Design review of the part built by this model. Coordinates are the model's own, in mm. A direction names the side the tool comes from. Give positions to 0.01 mm unless a question says otherwise; leave off trailing zeros. Order: outer loops, then holes, each group sorted by start corner. A loop starts at its lowest first (then second) coordinate and runs counter-clockwise, first axis right, second up. Notation, with made-up numbers: (-8.75, 82) -> (9.25, 82) arc R25 cw to (9.25, 119) -> close; hole circle Ø5 at (-1, 73.25). An arc over 180 degrees is marked (long way). Return JSON: item names as keys, results as strings.
```python
from build123d import *

# Parameters (mm, degrees)
SKETCH1_R           = 4.7625
SKETCH1_R_2         = 3.175
BOSS_EXTRUDE1_DEPTH = 8.3312
BOSS_EXTRUDE2_DEPTH = 8.3312
SKETCH3_R           = 2.0875
SKETCH3_R_2         = 1.5875
BOSS_EXTRUDE3_DEPTH = 8.3312
SKETCH4_R           = 2.0875
BOSS_EXTRUDE4_DEPTH = 0.001
SKETCH5_R           = 1.78
SKETCH5_R_2         = 1.28
BOSS_EXTRUDE5_DEPTH = 11.5062


with BuildPart() as part:
    # Sketch1 → Boss-Extrude1 (new body)
    with BuildSketch(Plane(origin=(0, 0, 0), x_dir=(1, 0, 0), z_dir=(0, 1, 0))):
        with Locations(Location((0, 0, 0), (0, 0, 270))):
            Circle(SKETCH1_R)
        with Locations(Location((0, 0, 0), (0, 0, 270))):
            Circle(SKETCH1_R_2, mode=Mode.SUBTRACT)
    extrude(amount=BOSS_EXTRUDE1_DEPTH)

    # Sketch2 → Boss-Extrude2 (add)
    with BuildSketch(Plane(origin=(0, 8.3312, 0), x_dir=(1, 0, 0), z_dir=(0, 1, 0))):
        Polygon((5.65061043, 0), (2.825305215, 4.893572179), (-2.825305215, 4.893572179), (-5.65061043, 0), (-2.825305215, -4.893572179), (2.825305215, -4.893572179), align=None)
    extrude(amount=BOSS_EXTRUDE2_DEPTH)

    # Sketch3 → Boss-Extrude3 (add)
    with BuildSketch(Plane(origin=(0, 16.6624, 0), x_dir=(1, 0, 0), z_dir=(0, 1, 0))):
        with Locations(Location((0, 0, 0), (0, 0, 270))):
            Circle(SKETCH3_R)
        with Locations(Location((0, 0, 0), (0, 0, 270))):
            Circle(SKETCH3_R_2, mode=Mode.SUBTRACT)
    extrude(amount=BOSS_EXTRUDE3_DEPTH)

    # Sketch4 → Boss-Extrude4 (add)
    with BuildSketch(Plane(origin=(0, 24.9936, 0), x_dir=(1, 0, 0), z_dir=(0, 1, 0))):
        with Locations(Location((0, 0, 0), (0, 0, 270))):
            Circle(SKETCH4_R)
    extrude(amount=BOSS_EXTRUDE4_DEPTH)

    # Sketch5 → Boss-Extrude5 (add)
    with BuildSketch(Plane.XY):
        with Locations(Location((0, 22.9946, 0), (0, 0, 180))):
            Circle(SKETCH5_R)
        with Locations(Location((0, 22.9946, 0), (0, 0, 180))):
            Circle(SKETCH5_R_2, mode=Mode.SUBTRACT)
    extrude(amount=BOSS_EXTRUDE5_DEPTH)


solid = part.part
```
Item 1: Machinability: for faces 5 (the face through (4.22, 12.44, 2.48)), 6 (the face through (0.027, 24.774, 0.606)), 7 (the face through (-0.821, 24.574, 6.225)), 8 (the face through (-1.93, 4.11, -2.52)), 9 (the face through (0, 12, 4.894)), which of the approach directions +Z, -Z, +X, -X, +Y, -Y give a long, thin tool a straight path to every point of the face, cutting with its end or side? Answer none if there is none.
Result set:
{"face 5": "+Z, +X, +Y, -Y", "face 6": "none", "face 7": "+Z", "face 8": "-Y", "face 9": "+Z, +X, -X, -Y"}
Item 2: Wall thickness on L1, parallel to Y at x = 0, z = 6.25; L2, parallel to X at y = 19.75, z = 0; L3, parallel to Y at x = 3, z = 1.75: over which ranges is each line inside the solid? List them lowest first. Write a range as [from, to].
Result set:
{"L1": "y = [21.21, 21.71], [24.27, 24.77]", "L2": "x = [-2.09, -1.59], [1.59, 2.09]", "L3": "y = [0, 16.66]"}
Item 3: Mouldability with a two-part tool opening along X and no side actions: class faces 1 (the face through (0.092, 20.77, -2.085)), 2 (the face through (-0.8, 24.2, 11.506)), 3 (the face through (0.277, 24.244, 6.508)), 4 (the face through (-1.22, 22.61, 0.61)) as released by +X, released by -X, zero draft, split by the parting line, or undercut.
Result set:
{"face 1": "split by the parting line", "face 2": "zero draft", "face 3": "undercut", "face 4": "undercut"}
Item 4: Add section D-D (z = -0.5). Give the boundary of the cut face in (x, y).
Result set:
{"outline": "(-5.36, 8.33) -> (-4.74, 8.33) -> (-4.74, 0) -> (-3.14, 0) -> (-3.14, 8.33) -> (3.14, 8.33) -> (3.14, 0) -> (4.74, 0) -> (4.74, 8.33) -> (5.36, 8.33) -> (5.36, 16.66) -> (2.03, 16.66) -> (2.03, 24.99) -> (-2.03, 24.99) -> (-2.03, 16.66) -> (-5.36, 16.66) -> close; hole (-1.51, 16.66) -> (1.51, 16.66) -> (1.51, 24.99) -> (-1.51, 24.99) -> close"}
Item 5: For pin 1 (1.5 mm diameter, centred on x = 0, y = 22.99, fed in from -Z); pin 2 (1.9 mm diameter, centred on x = 1.5, z = 0, fed in from -Y); pin 3 (4 mm diameter, centred on x = -2.5, y = 10, fed in from +Z), all flat-tipped, find the tip position at first contact; note any pin that passes through.
Result set:
{"pin 1": "stops at z = -2.09", "pin 2": "stops at y = 8.33", "pin 3": "stops at z = 4.89"}
Item 6: Add section A-A (z = 4.25). Give the boundary of the cut face in (x, y).
Result set:
{"outline": "(-3.2, 8.33) -> (-2.15, 8.33) -> (-2.15, 0) -> (2.15, 0) -> (2.15, 8.33) -> (3.2, 8.33) -> (3.2, 16.66) -> (-3.2, 16.66) -> close; circle Ø3.56 at (0, 22.99); hole circle Ø2.56 at (0, 22.99)"}
Item 7: Add section C-C (x = -3.75). Give the boundary of the cut face in (y, z).
Result set:
{"outline": "(0, -2.94) -> (8.33, -2.94) -> (8.33, -3.29) -> (16.66, -3.29) -> (16.66, 3.29) -> (8.33, 3.29) -> (8.33, 2.94) -> (0, 2.94) -> close"}
Item 8: Add section B-B (y = 17.75). Give the boundary of the cut face in (x, z) (1 decimal), plus the area to 3 significant figures.
Result set:
{"outline": "circle Ø4.2 at (0, 0); hole circle Ø3.2 at (0, 0)", "area": "5.77 mm^2"}
